Work out the finished part from the listing and answer in its coordinate system (mm). A direction names the side the tool comes from. Round coordinates to 2 decimals unless told otherwise and drop trailing zeros. Order: outer loops, then holes, each group sorted by start corner. A loop starts at its lowest first (then second) coordinate and runs counter-clockwise, first axis right, second up. Notation, with made-up numbers: M -31,-10.75 L -14,-10.75 A29 cw -14,15.25 Z; hole C -33.75,75.5 d3. An arc over 180 degrees is marked long. Return JSON: item names as keys, results as strings.
from build123d import *

# Parameters (mm, degrees)
F0_R     = 5.947106
F0_R_2   = 11.2
F1_DEPTH = 7


with BuildPart() as f1:
    # F0 (on Top) → F1 (new body)
    with BuildSketch(Plane.XY):
        with BuildLine():
            ThreePointArc((-12.799167, 7.407898), (-14.24174, 12.581914), (-18.153254, 16.263151))
            ThreePointArc((-18.153254, 16.263151), (-32.468011, 9.960046), (-23.128774, -2.586668))
            ThreePointArc((-23.128774, -2.586668), (-15.845609, 0.221242), (-12.799167, 7.407898))
        make_face()
        with Locations((-22.799167, 7.407898)):
            Circle(F0_R, mode=Mode.SUBTRACT)
        with BuildLine():
            ThreePointArc((9.857511, 22.29036), (9.964314, 23.1284), (10, 23.972463))
            ThreePointArc((10, 23.972463), (-1.401336, 33.873789), (-9.607252, 21.197447))
            ThreePointArc((-9.607252, 21.197447), (0.5606, 13.988189), (9.857511, 22.29036))
        make_face()
        with Locations((0, 23.972463)):
            Circle(F0_R, mode=Mode.SUBTRACT)
        with BuildLine():
            ThreePointArc((32.799167, 7.407898), (27.485316, 16.241924), (17.191166, 15.687411))
            ThreePointArc((17.191166, 15.687411), (13.476793, 3.789426), (24.245531, -2.48695))
            ThreePointArc((24.245531, -2.48695), (30.364339, 0.86816), (32.799167, 7.407898))
        make_face()
        with Locations((22.799167, 7.407898)):
            Circle(F0_R, mode=Mode.SUBTRACT)
        with BuildLine():
            ThreePointArc((24.09066, -19.39413), (23.074344, -15.001702), (20.231977, -11.502094))
            ThreePointArc((20.231977, -11.502094), (7.768516, -11.646195), (5.127051, -23.82738))
            ThreePointArc((5.127051, -23.82738), (16.367051, -29.131586), (24.09066, -19.39413))
        make_face()
        with Locations((14.09066, -19.39413)):
            Circle(F0_R, mode=Mode.SUBTRACT)
        with BuildLine():
            ThreePointArc((-4.09066, -19.39413), (-10.208766, -10.178334), (-21.076839, -12.239181))
            ThreePointArc((-21.076839, -12.239181), (-19.505734, -27.80109), (-4.687117, -22.796096))
            ThreePointArc((-4.687117, -22.796096), (-4.240903, -21.121059), (-4.09066, -19.39413))
        make_face()
        with Locations((-14.09066, -19.39413)):
            Circle(F0_R, mode=Mode.SUBTRACT)
        with BuildLine():
            ThreePointArc((9.857511, 22.29036), (0.5606, 13.988189), (-9.607252, 21.197447))
            ThreePointArc((-9.607252, 21.197447), (-14.222694, 19.323393), (-18.153254, 16.263151))
            ThreePointArc((-18.153254, 16.263151), (-14.24174, 12.581914), (-12.799167, 7.407898))
            ThreePointArc((-12.799167, 7.407898), (-15.845609, 0.221242), (-23.128774, -2.586668))
            ThreePointArc((-23.128774, -2.586668), (-22.772693, -7.555329), (-21.076839, -12.239181))
            ThreePointArc((-21.076839, -12.239181), (-10.208766, -10.178334), (-4.09066, -19.39413))
            ThreePointArc((-4.09066, -19.39413), (-4.240903, -21.121059), (-4.687117, -22.796096))
            ThreePointArc((-4.687117, -22.796096), (0.148396, -23.992843), (5.127051, -23.82738))
            ThreePointArc((5.127051, -23.82738), (7.768516, -11.646195), (20.231977, -11.502094))
            ThreePointArc((20.231977, -11.502094), (22.864407, -7.273064), (24.245531, -2.48695))
            ThreePointArc((24.245531, -2.48695), (13.476793, 3.789426), (17.191166, 15.687411))
            ThreePointArc((17.191166, 15.687411), (13.982585, 19.497843), (9.857511, 22.29036))
        make_face()
        Circle(F0_R_2, mode=Mode.SUBTRACT)
    extrude(amount=F1_DEPTH)


solid = f1.part
Item 1: Consider line 1 along Y through (x, z) = (0, 3); line 2 along Y through (x, z) = (3.5, 5.25); line 3 along X through (y, z) = (3.5, 1.75). Determine where each line is inside the solid, lowest interval first. Write a range as [from, to].
Output:
{"line 1": "y = [-23.98, -11.2], [11.2, 18.03], [29.92, 33.97]", "line 2": "y = [-24.03, -10.64], [10.64, 19.16], [28.78, 33.34]", "line 3": "x = [-32, -27.28], [-18.32, -10.64], [10.64, 18.32], [27.28, 32]"}
Item 2: Find section B-B (y = -21.5). Determine the outline of the cut face in (x, z), plus the area to 3 significant figures.
Output:
{"outline": "M -23.87,0 L -19.65,0 L -19.65,7 L -23.87,7 Z; M -8.53,0 L 8.53,0 L 8.53,7 L -8.53,7 Z; M 19.65,0 L 23.87,0 L 23.87,7 L 19.65,7 Z", "area": "178 mm^2"}
Item 3: Which of the six approach directions +Z, -Z, +X, -X, +Y, -Y give full straight-line access (tool end or side, diameter ignored) to faces 1 (the cylindrical face through (9.963, 23.117, 3.451)), 2 (the cylindrical face through (-14.865, -13.498, 3.451))?
Output:
{"face 1": "+Z, -Z, +X", "face 2": "+Z, -Z"}
Item 4: Find section A-A (x = -19). Determine the outline of the cut face in (y, z).
Output:
{"outline": "M -28.11,0 L -22.75,0 L -22.75,7 L -28.11,7 Z; M -16.04,0 L 2.83,0 L 2.83,7 L -16.04,7 Z; M 11.98,0 L 16.66,0 L 16.66,7 L 11.98,7 Z"}
Item 5: Find section D-D (y = 0). Determine the outline of the cut face in (x, z), plus the area to 3 significant figures.
Output:
{"outline": "M -29.52,0 L -11.2,0 L -11.2,7 L -29.52,7 Z; M 11.2,0 L 29.52,0 L 29.52,7 L 11.2,7 Z", "area": "256 mm^2"}
Item 6: Find section C-C (z = 6.25). Determine the outline of the cut face in (x, y).
Output:
{"outline": "M -23.13,-2.59 A18.12 ccw -21.08,-12.24 A10 ccw long -4.69,-22.8 A18.12 ccw 5.13,-23.83 A10 ccw 24.09,-19.39 A10 ccw 20.23,-11.5 A18.12 ccw 24.25,-2.49 A10 ccw 32.8,7.41 A10 ccw 17.19,15.69 A18.12 ccw 9.86,22.29 A10 ccw 10,23.97 A10 ccw long -9.61,21.2 A18.12 ccw -18.15,16.26 A10 ccw long Z; hole C -22.8,7.41 d11.89; hole C -14.09,-19.39 d11.89; hole C 0,0 d22.4; hole C 0,23.97 d11.89; hole C 14.09,-19.39 d11.89; hole C 22.8,7.41 d11.89"}
Item 7: Each of these flat-tipped pins is pushed along its axis until it touches: pin 1 (4 mm diameter, centred on x = 8.5, y = -0.5, fed in from -Z); pin 2 (12 mm diameter, centred on x = -5.5, y = 8.5, fed in from -Z); pin 3 (2 mm diameter, centred on x = 5.5, z = 5, fed in from -Y). Where does it stop, or does it pass through?
Output:
{"pin 1": "passes through", "pin 2": "stops at z = 0", "pin 3": "stops at y = -25.9"}
Item 8: The mould has two halves that part along X. Classify faces 3 (the cylindrical face through (22.836, -7.337, 3.451)), 4 (the cylindrical face through (-22.787, -7.487, 3.451)), 5 (the cylindrical face through (17.29, -14.38, 3.45)): pulls with the +X half, pulls with the -X half, needs draft (parallel to the pull), parting line crosses it, or undercut.
Output:
{"face 3": "pulls with the +X half", "face 4": "pulls with the -X half", "face 5": "undercut"}
